```python
from build123d import *

# Parameters (mm, degrees)
SKETCH1_W                      = 100
SKETCH1_H                      = 100
SKETCH1_W_2                    = 94
SKETCH1_H_2                    = 94
EXTRUDE_THIN1_DEPTH            = 130
FILLET1_R                      = 0.5
FILLET2_R                      = 3
F_8_0_8_DIAMETER_HOLE2_D       = 8
F_8_0_8_DIAMETER_HOLE3_D       = 8
F_10_0_10_DIAMETER_HOLE1_D     = 10
F_10_0_10_DIAMETER_HOLE2_D     = 10
F_21_0_21_DIAMETER_HOLE1_D     = 43
F_21_0_21_DIAMETER_HOLE1_DEPTH = 3
F_6_0_6_DIAMETER_HOLE1_D       = 6
F_6_0_6_DIAMETER_HOLE1_DEPTH   = 3
CUT_EXTRUDE1_REACH             = 173.464
SKETCH27_R                     = 2
SKETCH27_R_2                   = 3.5
CUT_EXTRUDE2_REACH             = 173.464
SKETCH31_R                     = 4
SKETCH34_R                     = 2
CUT_EXTRUDE3_DEPTH             = 10
SKETCH35_R                     = 2
CUT_EXTRUDE4_DEPTH             = 10
SKETCH36_R                     = 2
CUT_EXTRUDE5_DEPTH             = 10
SKETCH37_R                     = 2
CUT_EXTRUDE6_DEPTH             = 10
SKETCH38_R                     = 3.1
CUT_EXTRUDE7_DEPTH             = 10
SKETCH39_R                     = 3.1
CUT_EXTRUDE8_DEPTH             = 10


with BuildPart() as part:
    # Sketch1 → Extrude-Thin1 (new body)
    with BuildSketch(Plane.XY):
        Rectangle(SKETCH1_W, SKETCH1_H)
        Rectangle(SKETCH1_W_2, SKETCH1_H_2, mode=Mode.SUBTRACT)
    extrude(amount=EXTRUDE_THIN1_DEPTH)

    # Fillet1
    fillet1_edges = [part.edges().sort_by_distance(p)[0] for p in [
        (47, -47, 65),
        (47, 47, 65),
        (-47, 47, 65),
        (-47, -47, 65),
    ]]
    fillet(fillet1_edges, radius=FILLET1_R)

    # Fillet2
    fillet2_edges = [part.edges().sort_by_distance(p)[0] for p in [
        (50, -50, 65),
        (-50, -50, 65),
        (-50, 50, 65),
        (50, 50, 65),
    ]]
    fillet(fillet2_edges, radius=FILLET2_R)

    # Ø8.0 (8) Diameter Hole2 (through all)
    with Locations(Plane(origin=(0, 50, 0), x_dir=(1, 0, 0), z_dir=(0, 1, 0))):
        with Locations((28, -32), (28, -90)):
            Hole(F_8_0_8_DIAMETER_HOLE2_D / 2)

    # Ø8.0 (8) Diameter Hole3 (through all)
    with Locations(Plane(origin=(50, 0, 0), x_dir=(0, 0, -1), z_dir=(1, 0, 0))):
        with Locations((-14, 31), (-116, 31)):
            Hole(F_8_0_8_DIAMETER_HOLE3_D / 2)

    # Ø10.0 (10) Diameter Hole1 (through all)
    with Locations(Plane(origin=(0, 50, 0), x_dir=(1, 0, 0), z_dir=(0, 1, 0))):
        with Locations((-34, -56)):
            Hole(F_10_0_10_DIAMETER_HOLE1_D / 2)

    # Ø10.0 (10) Diameter Hole2 (through all)
    with Locations(Plane(origin=(50, 0, 0), x_dir=(0, 0, -1), z_dir=(1, 0, 0))):
        with Locations((-44, -31)):
            Hole(F_10_0_10_DIAMETER_HOLE2_D / 2)

    # Ø21.0 (21) Diameter Hole1
    with Locations(Plane(origin=(50, 0, 0), x_dir=(0, 0, -1), z_dir=(1, 0, 0))):
        with Locations((-70, 0)):
            Hole(F_21_0_21_DIAMETER_HOLE1_D / 2, depth=F_21_0_21_DIAMETER_HOLE1_DEPTH)

    # Ø6.0 (6) Diameter Hole1
    with Locations(Plane(origin=(50, 0, 0), x_dir=(0, 0, -1), z_dir=(1, 0, 0))):
        with Locations((-41.157258279, -16.652364697), (-53.347635303, 28.842741721), (-98.842741721, 16.652364697), (-86.652364697, -28.842741721)):
            Hole(F_6_0_6_DIAMETER_HOLE1_D / 2, depth=F_6_0_6_DIAMETER_HOLE1_DEPTH)

    # Sketch27 → Cut-Extrude1 (cut, up to next)
    with BuildSketch(Plane(origin=(50, 0, 0), x_dir=(0, 0, -1), z_dir=(1, 0, 0)), mode=Mode.PRIVATE) as cut_extrude1_sk1:
        with Locations(Location((-5, 13, 0), (0, 0, 90))):
            Circle(SKETCH27_R)
    cut_extrude1_tool1 = extrude(cut_extrude1_sk1.sketch, amount=-CUT_EXTRUDE1_REACH, mode=Mode.PRIVATE) & part.part
    # Sketch27 → Cut-Extrude1 (cut, up to next)
    with BuildSketch(Plane(origin=(50, 0, 0), x_dir=(0, 0, -1), z_dir=(1, 0, 0)), mode=Mode.PRIVATE) as cut_extrude1_sk2:
        with Locations(Location((-5, 4, 0), (0, 0, 90))):
            Circle(SKETCH27_R)
    cut_extrude1_tool2 = extrude(cut_extrude1_sk2.sketch, amount=-CUT_EXTRUDE1_REACH, mode=Mode.PRIVATE) & part.part
    # Sketch27 → Cut-Extrude1 (cut, up to next)
    with BuildSketch(Plane(origin=(50, 0, 0), x_dir=(0, 0, -1), z_dir=(1, 0, 0)), mode=Mode.PRIVATE) as cut_extrude1_sk3:
        with Locations(Location((-23, 8.5, 0), (0, 0, 90))):
            Circle(SKETCH27_R_2)
    cut_extrude1_tool3 = extrude(cut_extrude1_sk3.sketch, amount=-CUT_EXTRUDE1_REACH, mode=Mode.PRIVATE) & part.part
    # Sketch27 → Cut-Extrude1 (cut, up to next)
    with BuildSketch(Plane(origin=(50, 0, 0), x_dir=(0, 0, -1), z_dir=(1, 0, 0)), mode=Mode.PRIVATE) as cut_extrude1_sk4:
        with Locations(Location((-107, 8.5, 0), (0, 0, 270))):
            Circle(SKETCH27_R_2)
    cut_extrude1_tool4 = extrude(cut_extrude1_sk4.sketch, amount=-CUT_EXTRUDE1_REACH, mode=Mode.PRIVATE) & part.part
    # Sketch27 → Cut-Extrude1 (cut, up to next)
    with BuildSketch(Plane(origin=(50, 0, 0), x_dir=(0, 0, -1), z_dir=(1, 0, 0)), mode=Mode.PRIVATE) as cut_extrude1_sk5:
        with Locations(Location((-125, 4, 0), (0, 0, 270))):
            Circle(SKETCH27_R)
    cut_extrude1_tool5 = extrude(cut_extrude1_sk5.sketch, amount=-CUT_EXTRUDE1_REACH, mode=Mode.PRIVATE) & part.part
    # Sketch27 → Cut-Extrude1 (cut, up to next)
    with BuildSketch(Plane(origin=(50, 0, 0), x_dir=(0, 0, -1), z_dir=(1, 0, 0)), mode=Mode.PRIVATE) as cut_extrude1_sk6:
        with Locations(Location((-125, 13, 0), (0, 0, 270))):
            Circle(SKETCH27_R)
    cut_extrude1_tool6 = extrude(cut_extrude1_sk6.sketch, amount=-CUT_EXTRUDE1_REACH, mode=Mode.PRIVATE) & part.part
    add(cut_extrude1_tool1.solids().sort_by_distance((50, 13, 5))[0], mode=Mode.SUBTRACT)
    add(cut_extrude1_tool2.solids().sort_by_distance((50, 4, 5))[0], mode=Mode.SUBTRACT)
    add(cut_extrude1_tool3.solids().sort_by_distance((50, 8.5, 23))[0], mode=Mode.SUBTRACT)
    add(cut_extrude1_tool4.solids().sort_by_distance((50, 8.5, 107))[0], mode=Mode.SUBTRACT)
    add(cut_extrude1_tool5.solids().sort_by_distance((50, 4, 125))[0], mode=Mode.SUBTRACT)
    add(cut_extrude1_tool6.solids().sort_by_distance((50, 13, 125))[0], mode=Mode.SUBTRACT)

    # Sketch31 → Cut-Extrude2 (cut, up to next)
    with BuildSketch(Plane.ZY.offset(50), mode=Mode.PRIVATE) as cut_extrude2_sk1:
        with Locations(Location((14, -37, 0), (0, 0, 270))):
            Circle(SKETCH31_R)
    cut_extrude2_tool1 = extrude(cut_extrude2_sk1.sketch, amount=-CUT_EXTRUDE2_REACH, mode=Mode.PRIVATE) & part.part
    # Sketch31 → Cut-Extrude2 (cut, up to next)
    with BuildSketch(Plane.ZY.offset(50), mode=Mode.PRIVATE) as cut_extrude2_sk2:
        with Locations(Location((116, -37, 0), (0, 0, 270))):
            Circle(SKETCH31_R)
    cut_extrude2_tool2 = extrude(cut_extrude2_sk2.sketch, amount=-CUT_EXTRUDE2_REACH, mode=Mode.PRIVATE) & part.part
    add(cut_extrude2_tool1.solids().sort_by_distance((-50, -37, 14))[0], mode=Mode.SUBTRACT)
    add(cut_extrude2_tool2.solids().sort_by_distance((-50, -37, 116))[0], mode=Mode.SUBTRACT)

    # Sketch34 → Cut-Extrude3 (cut)
    with BuildSketch(Plane(origin=(0, 50, 0), x_dir=(1, 0, 0), z_dir=(0, 1, 0))):
        with Locations(Location((-22, -14, 0), (0, 0, 270))):
            Circle(SKETCH34_R)
        with Locations(Location((-11, -14, 0), (0, 0, 270))):
            Circle(SKETCH34_R)
        with Locations(Location((-11, -116, 0), (0, 0, 90))):
            Circle(SKETCH34_R)
        with Locations(Location((-22, -116, 0), (0, 0, 90))):
            Circle(SKETCH34_R)
    extrude(amount=-CUT_EXTRUDE3_DEPTH, mode=Mode.SUBTRACT)

    # Sketch35 → Cut-Extrude4 (cut)
    with BuildSketch(Plane.XZ.offset(50)):
        with Locations(Location((15, 44, 0), (0, 0, 270))):
            Circle(SKETCH35_R)
        with Locations(Location((4, 44, 0), (0, 0, 270))):
            Circle(SKETCH35_R)
    extrude(amount=-CUT_EXTRUDE4_DEPTH, mode=Mode.SUBTRACT)

    # Sketch36 → Cut-Extrude5 (cut)
    with BuildSketch(Plane.ZY.offset(50)):
        with Locations(Location((56, 19, 0), (0, 0, 270))):
            Circle(SKETCH36_R)
        with Locations(Location((56, 8, 0), (0, 0, 270))):
            Circle(SKETCH36_R)
    extrude(amount=-CUT_EXTRUDE5_DEPTH, mode=Mode.SUBTRACT)

    # Sketch37 → Cut-Extrude6 (cut)
    with BuildSketch(Plane(origin=(50, 0, 0), x_dir=(0, 0, -1), z_dir=(1, 0, 0))):
        with Locations(Location((-32, -17, 0), (0, 0, 90))):
            Circle(SKETCH37_R)
        with Locations(Location((-32, -6, 0), (0, 0, 90))):
            Circle(SKETCH37_R)
        with Locations(Location((-94, -6, 0), (0, 0, 90))):
            Circle(SKETCH37_R)
        with Locations(Location((-94, -17, 0), (0, 0, 90))):
            Circle(SKETCH37_R)
    extrude(amount=-CUT_EXTRUDE6_DEPTH, mode=Mode.SUBTRACT)

    # Sketch38 → Cut-Extrude7 (cut)
    with BuildSketch(Plane.XZ.offset(50)):
        with Locations(Location((38, 44, 0), (0, 0, 270))):
            Circle(SKETCH38_R)
        with Locations(Location((-19, 44, 0), (0, 0, 270))):
            Circle(SKETCH38_R)
    extrude(amount=-CUT_EXTRUDE7_DEPTH, mode=Mode.SUBTRACT)

    # Sketch39 → Cut-Extrude8 (cut)
    with BuildSketch(Plane.ZY.offset(50)):
        with Locations(Location((56, 35, 0), (0, 0, 270))):
            Circle(SKETCH39_R)
        with Locations(Location((56, -15, 0), (0, 0, 270))):
            Circle(SKETCH39_R)
    extrude(amount=-CUT_EXTRUDE8_DEPTH, mode=Mode.SUBTRACT)


solid = part.part
```
Part model, mm, in its own coordinate system. A direction names the side the tool comes from. Round coordinates to 2 decimals unless told otherwise and drop trailing zeros. Loops run counter-clockwise (first coordinate to the right, second up) from the corner with the lowest first, then second, coordinate; pieces in that order, holes last.
1. Drill centre lines: line 1 along Y through (x, z) = (-17, 65.5); line 2 along Y through (x, z) = (49, 125). Where is each one in solid material? Low to high.
Solutions:
line 1: y = -50 to -47, 47 to 50
line 2: y = -49.24 to 2, 6 to 11, 15 to 49.24
2. Two-plate mould, pull along Y, no slides. Class faces 1 (the face through (-50, -1, 64)), 2 (the face through (48.479, 32.201, 119.815)), 3 (the face through (-49.14, -49.1, 65.91)): pulls with the +Y half, pulls with the -Y half, needs draft (parallel to the pull), parting line crosses it, or undercut.
Solutions:
face 1: needs draft
face 2: undercut
face 3: pulls with the -Y half
3. Slice it at D-D (x = -42.5). Give the cut face in (y, z), and give its area (3 significant figures).
Solutions:
outline: (-50, 0) - (-47, 0) - (-47, 130) - (-50, 130) - close; (47, 0) - (50, 0) - (50, 130) - (47, 130) - close
area: 780 mm2
4. 3-axis set-ups, long thin cutter, end or side, ignore diameter. For faces 4 (the face through (-22, 49, 118)), 5 (the face through (49, 11, 5)), 6 (the face through (4, -49, 46)), 7 (the face through (47, -11, 50)), 8 (the face through (-48.521, 35.404, 59.074)): which of +Z, -Z, +X, -X, +Y, -Y reach the whole face in a straight line?
Solutions:
face 4: +Y
face 5: +X
face 6: -Y
face 7: +Z, -Z
face 8: -X
5. Slice it at B-B (z = 107). Give the cut face in (x, y), and give its area (3 significant figures).
Solutions:
outline: (-50, -47) arc R3 ccw to (-47, -50) - (47, -50) arc R3 ccw to (50, -47) - (50, 5) - (47, 5) - (47, -46.5) arc R0.5 cw to (46.5, -47) - (-46.5, -47) arc R0.5 cw to (-47, -46.5) - (-47, 46.5) arc R0.5 cw to (-46.5, 47) - (46.5, 47) arc R0.5 cw to (47, 46.5) - (47, 12) - (50, 12) - (50, 47) arc R3 ccw to (47, 50) - (-47, 50) arc R3 ccw to (-50, 47) - close
area: 1,140 mm2
6. Flat gauge pins, fed straight in: pin 1 (6.5 mm diameter, centred on x = 28, z = 90, fed in from -Y); pin 2 (3 mm diameter, centred on y = -17, z = 32, fed in from +X). Where does each tip first touch, or does it go through?
Solutions:
pin 1: passes through
pin 2: stops at x = -47
7. Slice it at C-C (y = -6). Give the cut face in (x, z), and give its area (3 significant figures).
Solutions:
outline: (-50, 0) - (-47, 0) - (-47, 130) - (-50, 130) - close; (47, 0) - (50, 0) - (50, 30) - (47, 30) - close; (47, 34) - (50, 34) - (50, 49.35) - (47, 49.35) - close; (47, 90.65) - (50, 90.65) - (50, 92) - (47, 92) - close; (47, 96) - (50, 96) - (50, 130) - (47, 130) - close
area: 632 mm2
8. Slice it at A-A (x = 15). Give the cut face in (y, z), and give its area (3 significant figures).
Solutions:
outline: (-50, 0) - (-47, 0) - (-47, 42) - (-50, 42) - close; (-50, 46) - (-47, 46) - (-47, 130) - (-50, 130) - close; (47, 0) - (50, 0) - (50, 130) - (47, 130) - close
area: 768 mm2
